Read the model definition and answer for the solid it produces. Units are mm, in the model's axes. A direction names the side the tool comes from. Coordinates: 2 decimals unless noted, no trailing zeros. Order: outer loops, then holes, each group sorted by start corner. A loop starts at its lowest first (then second) coordinate and runs counter-clockwise, first axis right, second up. Notation, with made-up numbers: M 39.5,9 L 55.5,9 A20 ccw 55.5,32 Z; hole C 75,-4.75 d1. An arc over 180 degrees is marked long. Write each question's results on one line, items separated by ' | '.
```python
from build123d import *

# Parameters (mm, degrees)
SKETCH1_R           = 18
BOSS_EXTRUDE1_DEPTH = 102
SKETCH2_R           = 1.5
CUT_EXTRUDE1_DEPTH  = 5
CIRPATTERN1_COUNT   = 4
SKETCH3_R           = 11
BOSS_EXTRUDE2_DEPTH = 3
SKETCH4_R           = 4
BOSS_EXTRUDE3_DEPTH = 17
CUT_EXTRUDE2_START  = -15
CUT_EXTRUDE2_DEPTH  = 15
BOSS_EXTRUDE4_DEPTH = 20


with BuildPart() as part:
    # Sketch1 → Boss-Extrude1 (new body)
    with BuildSketch(Plane(origin=(0, 0, 0), x_dir=(1, 0, 0), z_dir=(0, 1, 0))):
        with Locations(Location((0, 0, 0), (0, 0, 270))):
            Circle(SKETCH1_R)
    extrude(amount=BOSS_EXTRUDE1_DEPTH)

    # Sketch2 → Cut-Extrude1 (cut)
    with BuildSketch(Plane.XZ):
        with Locations(Location((-15, 0, 0), (0, 0, 270))):
            Circle(SKETCH2_R)
    cut_extrude1 = extrude(amount=-CUT_EXTRUDE1_DEPTH, mode=Mode.SUBTRACT)

    # CirPattern1: Cut-Extrude1 ×4 about axis
    cirpattern1_axis = Axis((0, 0, 0), (0, 1, 0))
    for i in range(1, CIRPATTERN1_COUNT):
        add(cut_extrude1.rotate(cirpattern1_axis, i * 360 / CIRPATTERN1_COUNT), mode=Mode.SUBTRACT)

    # Sketch3 → Boss-Extrude2 (add)
    with BuildSketch(Plane.XZ):
        with Locations(Location((0, 0, 0), (0, 0, 90))):
            Circle(SKETCH3_R)
    extrude(amount=BOSS_EXTRUDE2_DEPTH)

    # Sketch4 → Boss-Extrude3 (add)
    with BuildSketch(Plane.XZ.offset(3)):
        with Locations(Location((0, 0, 0), (0, 0, 270))):
            Circle(SKETCH4_R)
    extrude(amount=BOSS_EXTRUDE3_DEPTH)

    # Sketch5 → Cut-Extrude2 (cut)
    with BuildSketch(Plane.XZ.offset(20).offset(CUT_EXTRUDE2_START)):
        with BuildLine():
            Line((-2.645751311, -3), (2.645751311, -3))
            ThreePointArc((2.645751311, -3), (0, -4), (-2.645751311, -3))
        make_face()
    extrude(amount=CUT_EXTRUDE2_DEPTH, mode=Mode.SUBTRACT)

    # Sketch7 → Boss-Extrude4 (add)
    with BuildSketch(Plane(origin=(0, 102, 0), x_dir=(1, 0, 0), z_dir=(0, 1, 0))):
        with BuildLine():
            Line((-18, 0), (-18, -23))
            Line((-18, -23), (18, -23))
            Line((18, -23), (18, 0))
            ThreePointArc((18, 0), (0, 18), (-18, 0))
        make_face()
    extrude(amount=BOSS_EXTRUDE4_DEPTH)


solid = part.part
```
(1) Given pin 1 (8 mm diameter, centred on y = 47.5, z = -8, fed in from +X); pin 2 (2.5 mm diameter, centred on x = 0, z = 15, fed in from -Y); pin 3 (3 mm diameter, centred on y = 13, z = -13.5, fed in from -X), each flat-ended and moving along its own axis, determine where each tip first touches the part or whether it passes through.
Conclusion:
pin 1: x = 17.55 | pin 2: y = 5 | pin 3: x = -13.42
(2) The part is cut by section B-B, the plane z = 15. Write down the section's boundary in (x, y).
Conclusion:
outline: M -18,102 L -9.95,102 L -9.95,0 L -1.5,0 L -1.5,5 L 1.5,5 L 1.5,0 L 9.95,0 L 9.95,102 L 18,102 L 18,122 L -18,122 Z
(3) For faces 5 (the flat face through (0, -12, -3)), 6 (the flat face through (-8, 0, -8)), 7 (the flat face through (0, 102, 19)), 8 (the flat face through (0, 112, 23)), determine the directions among +Z, -Z, +X, -X, +Y, -Y from which every point of the face is accessible in a straight line to the end or side of a thin tool.
Conclusion:
face 5: -Z, +X, -X, -Y | face 6: -Y | face 7: +Z, -Y | face 8: +Z, +X, -X, +Y, -Y
(4) The part is cut by section C-C, the plane y = 50.5. Write down the section's boundary in (x, z), then the cut area to 3 significant figures.
Conclusion:
outline: C 0,0 d36 | area: 1,020 mm²
(5) The part is cut by section D-D, the plane x = 5.5. Write down the section's boundary in (y, z).
Conclusion:
outline: M -3,-9.53 L 0,-9.53 L 0,-17.14 L 122,-17.14 L 122,23 L 102,23 L 102,17.14 L 0,17.14 L 0,9.53 L -3,9.53 Z
(6) The part is cut by section A-A, the plane x = 0. Write down the section's boundary in (y, z).
Conclusion:
outline: M -20,-3 L -5,-3 L -5,-4 L -3,-4 L -3,-11 L 0,-11 L 0,-13.5 L 5,-13.5 L 5,-16.5 L 0,-16.5 L 0,-18 L 122,-18 L 122,23 L 102,23 L 102,18 L 0,18 L 0,16.5 L 5,16.5 L 5,13.5 L 0,13.5 L 0,11 L -3,11 L -3,4 L -20,4 Z
(7) Straight lines are drawn through the part: line 1 (Z direction, x = 0, y = 1.9); line 2 (Y direction, x = -2.5, z = -15). For each, find the intervals that lie inside material, in ascending order.
Conclusion:
line 1: -18 to -16.5, -13.5 to 13.5, 16.5 to 18 | line 2: 0 to 122
(8) The mould has two halves that part along X. Classify faces 1 (the flat face through (15, 5, 0)), 2 (the flat face through (0, -20, 1)), 3 (the cylindrical face through (-14.55, 2.46, -1.43)), 4 (the cylindrical face through (0.791, 60.146, -17.983)): pulls with the +X half, pulls with the -X half, needs draft (parallel to the pull), parting line crosses it, or undercut.
Conclusion:
face 1: undercut | face 2: needs draft | face 3: undercut | face 4: parting line crosses it
